Print and shaded views of the part. All mm, measured from the part's lowest x, y and z. A direction names the side the tool comes from. Round coordinates to 2 decimals unless told otherwise and drop trailing zeros. Loops run counter-clockwise (first coordinate to the right, second up) from the corner with the lowest first, then second, coordinate; pieces in that order, holes last. Notation, with made-up numbers: (0, 31.5) - (31, 31.5) arc R15 ccw to (31, 51.5) - close; hole circle Ø7 at (64.25, -20). An arc over 180 degrees is marked (long way). Use one line per item in the form item = value.
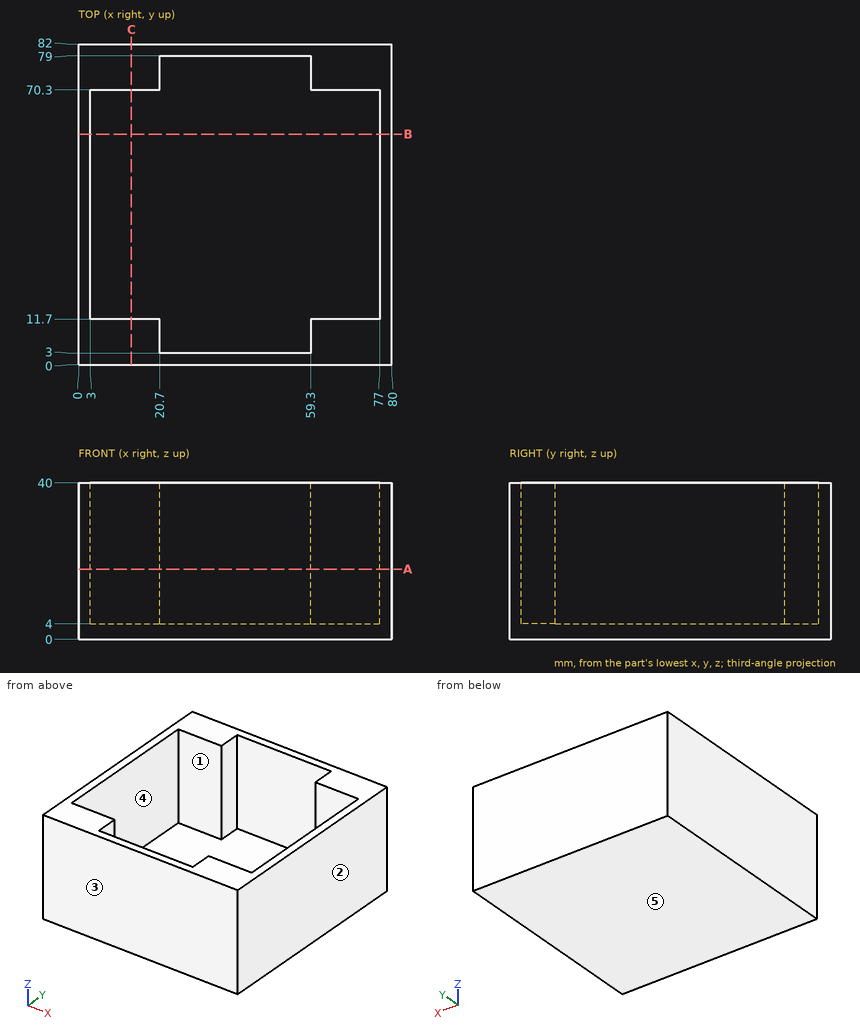
1) Slice it at B-B (y = 59). Write the cut outline in (x, z), plus the area to 3 significant figures.
Report:
outline = (0, 0) - (80, 0) - (80, 40) - (77, 40) - (77, 4) - (3, 4) - (3, 40) - (0, 40) - close
area = 536 mm^2
2) Drill centre lines: probe 1 along Y at (x, z) = (48.5, 7); probe 2 along X at (y, z) = (68, 17); probe 3 along X at (y, z) = (75, 33). Where is each one in solid material? Low to high.
Report:
probe_1 = 0 to 3, 79 to 82
probe_2 = 0 to 3, 77 to 80
probe_3 = 0 to 20.7, 59.3 to 80
3) Slice it at C-C (x = 13.5). Write the cut outline in (y, z), plus the area to 3 significant figures.
Report:
outline = (0, 0) - (82, 0) - (82, 40) - (70.3, 40) - (70.3, 4) - (11.7, 4) - (11.7, 40) - (0, 40) - close
area = 1,170 mm^2
4) Slice it at A-A (z = 18). Write the cut outline in (x, y), plus the area to 3 significant figures.
Report:
outline = (0, 0) - (80, 0) - (80, 82) - (0, 82) - close; hole (3, 11.7) - (20.7, 11.7) - (20.7, 3) - (59.3, 3) - (59.3, 11.7) - (77, 11.7) - (77, 70.3) - (59.3, 70.3) - (59.3, 79) - (20.7, 79) - (20.7, 70.3) - (3, 70.3) - close
area = 1,550 mm^2
5) Tool access for the marked faces 1 and 2: list every direction of +Z, -Z, +X, -X, +Y, -Y with a clear straight run to the whole face (end or side of a thin tool).
Report:
face_1 = +Z
face_2 = +Z, -Z, +X, +Y, -Y
6) Two-plate mould, pull along Y, no slides. Class the marked faces 3, 4 and 5: +Y half, -Y half, draft (parallel to the pull), parting line (faces both ways), or undercut.
Report:
face_3 = -Y half
face_4 = undercut
face_5 = draft
